from build123d import *

# Parameters (mm, degrees)
SKETCH_1_RX         = 19
SKETCH_1_RY         = 5
EXTRUDE_1_DEPTH     = 1
SKETCH_2_R          = 2.5
EXTRUDE_2_DEPTH     = 3
SKETCH_3_R          = 1
CUT_EXTRUDE_1_DEPTH = 5
SKETCH_4_R          = 2
CUT_EXTRUDE_2_DEPTH = 3
SKETCH_5_R          = 1.5
CUT_EXTRUDE_3_DEPTH = 3
SKETCH_6_R          = 2.5
SKETCH_6_R_2        = 2
EXTRUDE_3_DEPTH     = 1


with BuildPart() as part:
    # 스케치1 → 보스-돌출1 (new body)
    with BuildSketch(Plane.XY):
        with Locations(Location((0, 0), (0, 0, 180))):
            Ellipse(SKETCH_1_RX, SKETCH_1_RY)
    extrude(amount=EXTRUDE_1_DEPTH)

    # 스케치2 → 보스-돌출2 (add)
    with BuildSketch(Plane.XY.offset(1)):
        Circle(SKETCH_2_R)
    extrude(amount=EXTRUDE_2_DEPTH)

    # 스케치3 → 컷-돌출1 (cut, through all)
    with BuildSketch(Plane(origin=(0, 0, 0), x_dir=(-1, 0, 0), z_dir=(0, 0, -1))):
        with Locations((-5, 0)):
            Circle(SKETCH_3_R)
        with Locations((-8, 0)):
            Circle(SKETCH_3_R)
        with Locations((-11, 0)):
            Circle(SKETCH_3_R)
        with Locations((-14, 0)):
            Circle(SKETCH_3_R)
        with Locations((14, 0)):
            Circle(SKETCH_3_R)
        with Locations((11, 0)):
            Circle(SKETCH_3_R)
        with Locations((8, 0)):
            Circle(SKETCH_3_R)
        with Locations((5, 0)):
            Circle(SKETCH_3_R)
    extrude(amount=-CUT_EXTRUDE_1_DEPTH, mode=Mode.SUBTRACT)

    # 스케치4 → 컷-돌출2 (cut)
    with BuildSketch(Plane.XY.offset(4)):
        Circle(SKETCH_4_R)
    extrude(amount=-CUT_EXTRUDE_2_DEPTH, mode=Mode.SUBTRACT)

    # 스케치5 → 컷-돌출3 (cut)
    with BuildSketch(Plane(origin=(0, 0, 0), x_dir=(-1, 0, 0), z_dir=(0, 0, -1))):
        Circle(SKETCH_5_R)
    extrude(amount=-CUT_EXTRUDE_3_DEPTH, mode=Mode.SUBTRACT)

    # 스케치6 → 보스-돌출3 (add)
    with BuildSketch(Plane(origin=(0, 0, 0), x_dir=(-1, 0, 0), z_dir=(0, 0, -1))):
        Circle(SKETCH_6_R)
        Circle(SKETCH_6_R_2, mode=Mode.SUBTRACT)
    extrude(amount=EXTRUDE_3_DEPTH)


solid = part.part
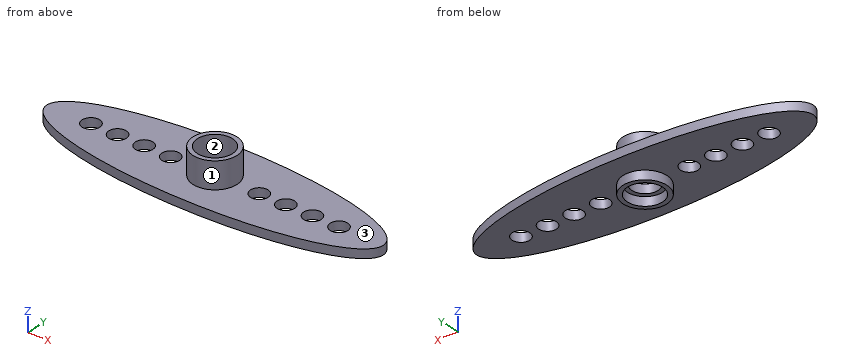
For this review, take the finished solid that the model builds, in its own axes (mm). Face numbers are marked on the shaded views. Round coordinates to 2 decimals unless told otherwise and drop trailing zeros. Loops run counter-clockwise (first coordinate to the right, second up) from the corner with the lowest first, then second, coordinate; pieces in that order, holes last. Notation, with made-up numbers: (61, -21) - (81, -21) arc R14 cw to (81, 6) - close; hole circle Ø10 at (-13, 21.25). An arc over 180 degrees is marked (long way). Put each result on its own line as item: value. Start each with the question number.
1. For probe 1 along Y at (x, z) = (0, 0.3); probe 2 along Y at (x, z) = (0, 2.2); probe 3 along Z at (x, y) = (-4, -2.75), list the stretches that pass through material, from the lowest coordinate up. Write a range as [from, to].
2. Mouldability with a two-part tool opening along X and no side actions: class the marked faces 1, 2 and 3 as +X half, -X half, draft (parallel to the pull), parting line (faces both ways), or undercut.
3. Consider section A-A on y = 0. State how many separate pieces and enclosed holes the cut face has, plus the area to 3 significant figures.
4. Insertion check: P1, Ø2.5, axis at x = -14, y = 0, coming from the +Z side; P2, Ø2, axis at x = -3.5, z = 0.5, coming from the +Y side; P3, Ø3, axis at x = 10.5, z = -0.5, coming from the -Y side. Each pin has a flat end and moves straight along its axis. Give the tip position at first contact, or say it passes through.
5. Consider section B-B on z = 3.5. State the section outline as (x, y) points.
Result sheet:
1. probe 1: [-5, -1.5], [1.5, 5]
1. probe 2: [-2.5, -2], [2, 2.5]
1. probe 3: [0, 1]
2. face 1: parting line
2. face 2: undercut
2. face 3: draft
3. separate pieces: 10
3. enclosed holes: 0
3. area: 23.0 mm^2
4. P1: z = 1
4. P2: y = 4.96
4. P3: y = -4.39
5. outline: circle Ø5 at (0, 0); hole circle Ø4 at (0, 0)
